Could you check a few things on this model? Use its own coordinates, in mm. Face numbers are marked on the shaded views. A direction names the side the tool comes from. Give positions to 0.01 mm unless a question says otherwise; leave off trailing zeros. Order: outer loops, then holes, each group sorted by start corner. A loop starts at its lowest first (then second) coordinate and runs counter-clockwise, first axis right, second up. Notation, with made-up numbers: M -14.5,-8 L 23.5,-8 A16 cw 23.5,-3 Z; hole C 68.5,17 d1. An arc over 180 degrees is marked long. Use a Markdown table: item, result. Add a question column.
Item 1: I'm going to push a flat-ended pin straight in: pin 1 Ø1.2 at (x, z) = (-1.5, -3.5) entering from -Y. Where does the tip first touch, or does it pass through?
Item 2: Suppose I cut it at D-D on z = -6.75. Write out the boundary of the cut face in (x, y).
Item 3: For the marked faces 1, 2 and 3, which set-ups out of +Z, -Z, +X, -X, +Y, -Y let a thin tool reach every point of the face, with its end or its side?
Item 4: Suppose I cut it at B-B on x = -2. Write out the boundary of the cut face in (y, z).
Item 5: If I drill on L1, parallel to X at y = 1, z = -2; L2, parallel to X at y = 4, z = -5, over which ranges is the centre line in solid material (lowest first)? Write a range as from..to.
Item 6: If we mould it in two halves opening along Z, with no side actions, what happens to the marked faces 4, 5, 6 and 7? For each: released by +Z, released by -Z, zero draft, split by the parting line, or undercut.
Item 7: Suppose I cut it at A-A on y = 1.5. Write out the boundary of the cut face in (x, z), plus the area to 3 significant figures.
Item 8: Suppose I cut it at C-C on z = -4. Write out the boundary of the cut face in (x, y), plus the area to 3 significant figures.
from build123d import *

# Parameters (mm, degrees)
SKETCH1_W           = 8
SKETCH1_H           = 15
BOSS_EXTRUDE1_DEPTH = 3
SKETCH2_W           = 17
SKETCH2_H           = 8
SKETCH2_R           = 1
BOSS_EXTRUDE2_DEPTH = 3
SKETCH3_W           = 4
SKETCH3_H           = 8
SKETCH3_R           = 1
BOSS_EXTRUDE3_DEPTH = 3


with BuildPart() as part:
    # Sketch1 → Boss-Extrude1 (new body)
    with BuildSketch(Plane(origin=(0, 0, 0), x_dir=(0, 0, -1), z_dir=(1, 0, 0))):
        with Locations((4, 7.5)):
            Rectangle(SKETCH1_W, SKETCH1_H)
    extrude(amount=BOSS_EXTRUDE1_DEPTH)

    # Sketch2 → Boss-Extrude2 (add)
    with BuildSketch(Plane(origin=(0, 0, 0), x_dir=(1, 0, 0), z_dir=(0, 1, 0))):
        with Locations((11.5, 4)):
            Rectangle(SKETCH2_W, SKETCH2_H)
        with Locations(Location((17, 4, 0), (0, 0, 270))):
            Circle(SKETCH2_R, mode=Mode.SUBTRACT)
    extrude(amount=BOSS_EXTRUDE2_DEPTH)

    # Sketch3 → Boss-Extrude3 (add)
    with BuildSketch(Plane(origin=(0, 15, 0), x_dir=(1, 0, 0), z_dir=(0, 1, 0))):
        with Locations((-2, 4)):
            Rectangle(SKETCH3_W, SKETCH3_H)
        with Locations(Location((-2, 3.81772143, 0), (0, 0, 270))):
            Circle(SKETCH3_R, mode=Mode.SUBTRACT)
    extrude(amount=-BOSS_EXTRUDE3_DEPTH)


solid = part.part
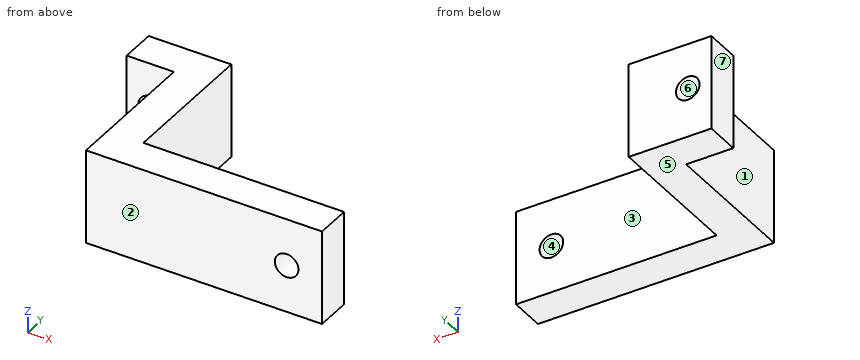
Findings below:
| question | item | result |
|---|---|---|
| 1 | pin 1 | stops at y = 12 |
| 2 | outline | M -4,12 L 0,12 L 0,0 L 20,0 L 20,3 L 3,3 L 3,15 L -4,15 Z |
| 3 | face 1 | +Z, -Z, -X, -Y |
| 3 | face 2 | +Z, -Z, +X, -X, -Y |
| 3 | face 3 | +Z, -Z, +X, +Y |
| 4 | outline | M 12,-8 L 15,-8 L 15,-4.82 L 12,-4.82 Z; M 12,-2.82 L 15,-2.82 L 15,0 L 12,0 Z |
| 5 | L1 | x = 0..20 |
| 5 | L2 | x = 0..3 |
| 6 | face 4 | undercut |
| 6 | face 5 | released by -Z |
| 6 | face 6 | undercut |
| 6 | face 7 | zero draft |
| 7 | outline | M 0,-8 L 20,-8 L 20,0 L 0,0 Z; hole C 17,-4 d2 |
| 7 | area | 157 mm^2 |
| 8 | outline | M -4,12 L -2.98,12 L -2.98,15 L -4,15 Z; M -1.02,12 L 0,12 L 0,0 L 16,0 L 16,3 L 3,3 L 3,15 L -1.02,15 Z; M 18,0 L 20,0 L 20,3 L 18,3 Z |
| 8 | area | 96.1 mm^2 |
